```python
from build123d import *

# Parameters (mm, degrees)
BOSS_EXTRUDE1_DEPTH = 1.905
CHAMFER1_SIZE       = 0.762


with BuildPart() as part:
    # Sketch1 → Boss-Extrude1 (new body)
    with BuildSketch(Plane(origin=(0, 0, 0), x_dir=(1, 0, 0), z_dir=(0, 1, 0))):
        with BuildLine():
            ThreePointArc((10.16, 0), (-6.72020833, 7.62), (-1.27, -10.080312495))
            Line((-1.27, -10.080312495), (-1.27, -1.82389864))
            ThreePointArc((-1.27, -1.82389864), (-1.028817586, 1.970035691), (2.2225, 0))
            ThreePointArc((2.2225, 0), (1.970035691, -1.028817586), (1.27, -1.82389864))
            Line((1.27, -1.82389864), (1.27, -10.080312495))
            ThreePointArc((1.27, -10.080312495), (7.62, -6.72020833), (10.16, 0))
        make_face()
    extrude(amount=BOSS_EXTRUDE1_DEPTH)

    # Chamfer1
    chamfer1_edges = [part.edges().sort_by_distance(p)[0] for p in [
        (0, 1.905, -10.16),
    ]]
    chamfer(chamfer1_edges, length=CHAMFER1_SIZE)


solid = part.part
```
Build history of the part. All positions in model axes, mm. A direction names the side the tool comes from. Coordinates: 2 decimals unless noted, no trailing zeros. Order: outer loops, then holes, each group sorted by start corner. A loop starts at its lowest first (then second) coordinate and runs counter-clockwise, first axis right, second up.
Item 1: Drop flat-ended pins along their axis: pin 1 Ø2 at (x, z) = (0, 0) entering from +Y; pin 2 Ø1 at (y, z) = (1, 6.5) entering from +X. Give the stop position or say it passes through.
Filled in:
pin 1: passes through
pin 2: stops at x = 8.2
Item 2: Saw through at B-B on x = 0. List the corners of the cut face in (y, z) (1 decimal), then the cut area to 3 significant figures.
Filled in:
outline: (0, -10.2) - (1.1, -10.2) - (1.9, -9.4) - (1.9, -2.2) - (0, -2.2) - close
area: 14.8 mm2
Item 3: Saw through at A-A on y = 0.55. List the corners of the cut face in (x, z) (1 decimal).
Filled in:
outline: (-1.3, 1.8) - (-1.3, 10.1) arc R10.2 ccw (long way) to (1.3, 10.1) - (1.3, 1.8) arc R2.2 cw (long way) to start
Item 4: Drill centre lines: L1, parallel to X at y = 0.8, z = 0; L2, parallel to X at y = 1, z = 3.5; L3, parallel to Z at x = 2, y = 1.75. Where is each one in solid material? Low to high.
Filled in:
L1: x = -10.16 to -2.22, 2.22 to 10.16
L2: x = -9.54 to -1.27, 1.27 to 9.54
L3: z = -9.34 to -0.97, 0.97 to 9.34
Item 5: Tool access for faces 4 (the flat face through (2, 1.905, -2)), 5 (the flat face through (1.27, 1, 6)): list every direction of +Z, -Z, +X, -X, +Y, -Y with a clear straight run to the whole face (end or side of a thin tool).
Filled in:
face 4: +Z, -Z, +X, -X, +Y
face 5: +Z, +Y, -Y
Item 6: Mould opens along X. For faces 1 (the flat face through (-1.27, 1, 6)), 2 (the cylindrical face through (0.43, 0.56, -10.15)), 3 (the flat face through (-0.1, 0, -2.4)) say: released by +X, released by -X, zero draft, split by the parting line, or undercut.
Filled in:
face 1: undercut
face 2: split by the parting line
face 3: zero draft
